Could you check a few things on this model? Use its own coordinates, in mm. Round coordinates to 2 decimals unless told otherwise and drop trailing zeros. Write each loop counter-clockwise with the first axis right and the second up, starting at its lowest first coordinate (ties: lowest second). Pieces come first, ordered by that corner, then holes. Notation, with made-up numbers: (34, 47) - (88, 47) arc R20 ccw to (88, 57) - close; hole circle Ø4 at (32, -4). An arc over 180 degrees is marked (long way). Write each question's results on one line, items separated by ' | '. Start each with the question number.
(1) Imagine slicing it at C-C on x = 4.25. Write out the boundary of the cut face in (y, z), then the cut area to 3 significant figures.
(2) For P1, Ø2, axis at y = 0, z = 0, coming from the +X side; P2, Ø3, axis at x = -6.5, y = 2, coming from the +Z side; P3, Ø1, axis at x = 2.5, y = -1, coming from the -Z side, each with a flat end and sliding along its axis, tell me the tip position at first contact or that it passes through.
(3) Imagine slicing it at A-A on z = 0. Write out the boundary of the cut face in (x, y).
(4) Please list where these lines run through material, in increasing order: line 1 (Z direction, x = 2.75, y = 0); line 2 (Y direction, x = -10, z = 0.75). Write a range as [from, to].
(5) Thinking about a two-plate mould opening in Z: for faces 1 (the cylindrical face through (0.15, -0.54, -2.44)), 2 (the cylindrical face through (-0.15, -0.17, -1.29)), 3 (the flat face through (11, 0, -2)), which applies, +Z half, -Z half, draft (parallel to the pull), parting line (faces both ways), or undercut?
Autodesk Inventor part; units mm, degrees
ref_plane "YZ Plane" through (0, 0, 0) normal (1, 0, 0) x (0, 1, 0)
ref_plane "XZ Plane" through (0, 0, 0) normal (0, 1, 0) x (-1, 0, 0)
ref_plane "XY Plane" through (0, 0, 0) normal (0, 0, 1) x (1, 0, 0)
sketch "スケッチ1" plane through (0, 0, 0) normal (1, 0, 0) x (0, 1, 0)
  circle A0 centre (0, 0) radius 2.5
  circle A1 centre (0, 0) radius 1.3
  dimension "d0" = 5
  dimension "d1" = 2.6
extrude "押し出し1" add sketch "スケッチ1" along normal mid plane 22
chamfer "面取り1" distance 0.2 angle 45 4 edges at (11, -1.3, 0) (11, -2.5, 0) (-11, -1.3, 0) (-11, -2.5, 0)
properties part number "AR-2622"
Response:
1) outline: circle Ø5 at (0, 0); hole circle Ø2.6 at (0, 0) | area: 14.3 mm²
2) P1: through | P2: z = 2.45 | P3: z = -2.45
3) outline: (-11, -2.3) - (-10.8, -2.5) - (10.8, -2.5) - (11, -2.3) - (11, -1.5) - (10.8, -1.3) - (-10.8, -1.3) - (-11, -1.5) - close; (-11, 1.5) - (-10.8, 1.3) - (10.8, 1.3) - (11, 1.5) - (11, 2.3) - (10.8, 2.5) - (-10.8, 2.5) - (-11, 2.3) - close
4) line 1: [-2.5, -1.3], [1.3, 2.5] | line 2: [-2.38, -1.06], [1.06, 2.38]
5) face 1: parting line | face 2: undercut | face 3: draft
